Check sheet for the drawn part. Datum: minimum x, y, z corner. Units: mm. A direction names the side the tool comes from. Coordinates: 2 decimals unless noted, no trailing zeros. Write each loop counter-clockwise with the first axis right and the second up, starting at its lowest first coordinate (ties: lowest second). Pieces come first, ordered by that corner, then holes. Notation, with made-up numbers: (-32.5, 77) -> (-13.5, 77) arc R10 ccw to (-13.5, 82) -> close; hole circle Ø2 at (74, -16.5). An arc over 180 degrees is marked (long way). Write item = value, one per line. Start each with the question number.
(1) Section check A-A (x = 3). Record the cut outline in (y, z).
(2) Set-up check for the marked faces 1 and 2: record each of +Z, -Z, +X, -X, +Y, -Y from which the full face is reachable in a straight line by a thin tool's end or side.
(3) Material ranges on probe 1 along Z at (x, y) = (0.6, 2.7); probe 2 along Z at (x, y) = (4.6, 2.2); probe 3 along Y at (x, z) = (3.5, 1.5), recorded low to high. Write a range as [from, to].
(4) Gauge pin test, flat ends, axial feed: pin 1 Ø2 at (x, y) = (3.5, 2.5) entering from -Z; pin 2 Ø1.5 at (x, y) = (3.5, 0.5) entering from -Z; pin 3 Ø3 at (y, z) = (4.5, 15) entering from +X; pin 4 Ø1 at (x, z) = (1.5, 5.5) entering from -Y. Record the tip position at first contact, or that the pin passes through.
(5) Section check C-C (z = 6.25). Record the cut outline in (x, y), plus the area to 3 significant figures.
(6) Section check D-D (y = 1.3). Record the cut outline in (x, z), plus the area to 3 significant figures.
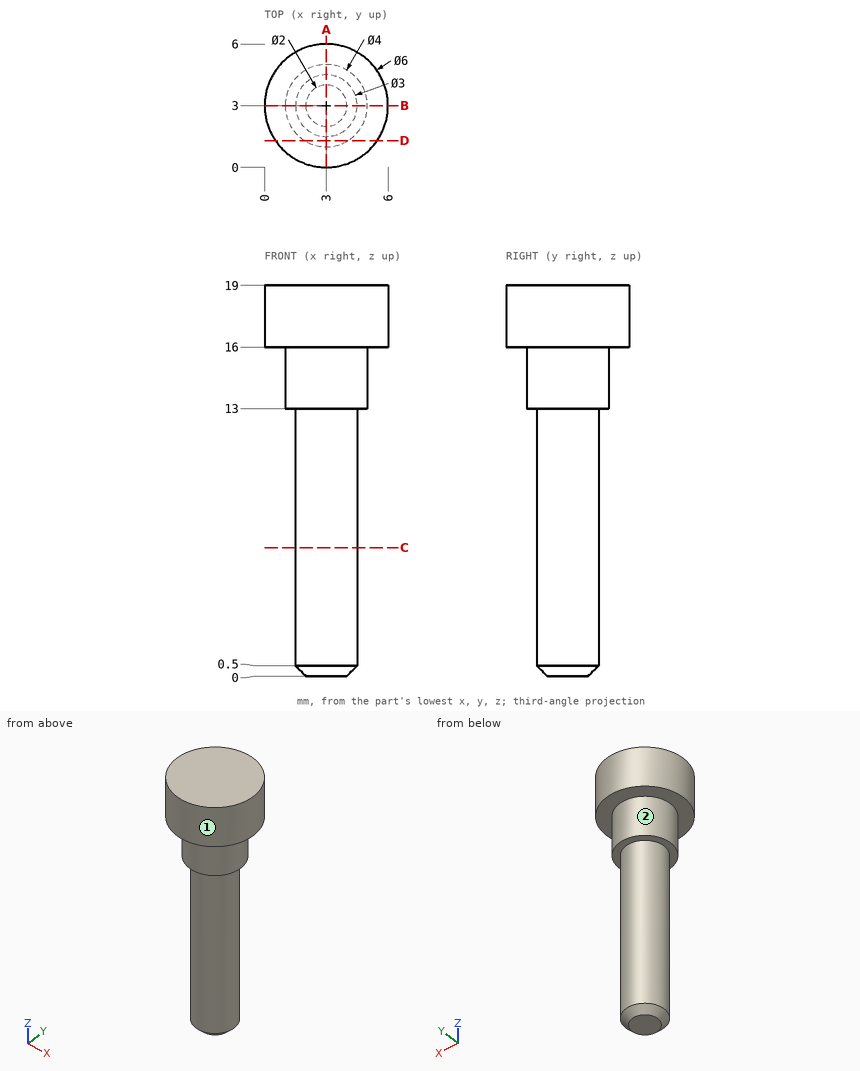
Response:
q1.outline = (0, 16) -> (1, 16) -> (1, 13) -> (1.5, 13) -> (1.5, 0.5) -> (2, 0) -> (4, 0) -> (4.5, 0.5) -> (4.5, 13) -> (5, 13) -> (5, 16) -> (6, 16) -> (6, 19) -> (0, 19) -> close
q2.face_1 = +Z, -Z
q2.face_2 = -Z
q3.probe_1 = [16, 19]
q3.probe_2 = [13, 19]
q3.probe_3 = [1.59, 4.41]
q4.pin_1 = 0
q4.pin_2 = 13
q4.pin_3 = 5.98
q4.pin_4 = 1.88
q5.outline = circle Ø3 at (3, 3)
q5.area = 7.07 mm2
q6.outline = (0.53, 16) -> (1.95, 16) -> (1.95, 13) -> (4.05, 13) -> (4.05, 16) -> (5.47, 16) -> (5.47, 19) -> (0.53, 19) -> close
q6.area = 21.2 mm2
